```python
from build123d import *

# Parameters (mm, degrees)
SKETCH1_R           = 15
BOSS_EXTRUDE1_DEPTH = 10
SKETCH2_R           = 3.75
CUT_EXTRUDE1_DEPTH  = 5
SKETCH3_R           = 3.75
CUT_EXTRUDE2_DEPTH  = 24.452078799


with BuildPart() as part:
    # Sketch1 → Boss-Extrude1 (new body)
    with BuildSketch(Plane(origin=(0, 0, 0), x_dir=(1, 0, 0), z_dir=(0, 1, 0))):
        with Locations(Location((0, 0, 0), (0, 0, 270))):
            Circle(SKETCH1_R)
    extrude(amount=BOSS_EXTRUDE1_DEPTH)

    # Sketch2 → Cut-Extrude1 (cut)
    with BuildSketch(Plane.XZ):
        with Locations(Location((0, 0, 0), (0, 0, 270))):
            Circle(SKETCH2_R)
    extrude(amount=-CUT_EXTRUDE1_DEPTH, mode=Mode.SUBTRACT)

    # Sketch3 → Cut-Extrude2 (cut, through all)
    with BuildSketch(Plane(origin=(0, 10, 0), x_dir=(1, 0, 0), z_dir=(0, 1, 0))):
        with Locations(Location((0, 0, 0), (0, 0, 90))):
            Circle(SKETCH3_R)
    extrude(amount=-CUT_EXTRUDE2_DEPTH, mode=Mode.SUBTRACT)


solid = part.part
```
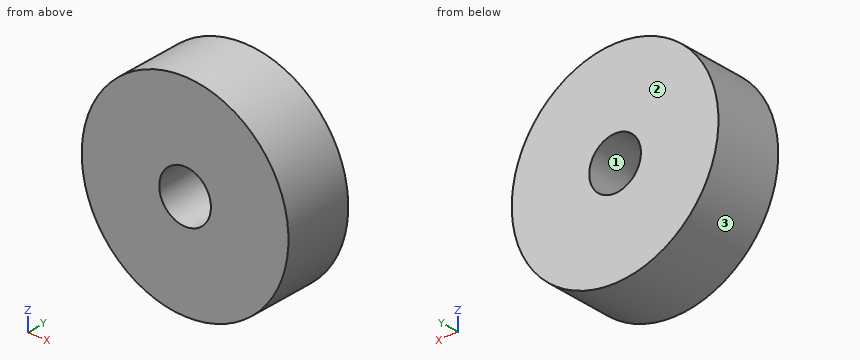
Input: part model. Units: mm. Frame: model coordinates. Face numbers are marked on the shaded views. Give positions to 0.01 mm unless a question says otherwise; leave off trailing zeros. Order: outer loops, then holes, each group sorted by start corner. A loop starts at its lowest first (then second) coordinate and runs counter-clockwise, first axis right, second up. Notation, with made-up numbers: (-22, -16.5) - (-2, -16.5) arc R17 cw to (-2, 16.5) - close; hole circle Ø4 at (85.5, -30). An arc over 180 degrees is marked (long way). Use a Markdown table: item, result.
(1) Line query: line 1 (X direction, y = 3, z = 0); line 2 (X direction, y = 9, z = 1.75); line 3 (X direction, y = 9.5, z = 4.25). Output: solid intervals per line, ascending. Write a range as from..to.
Computed values:
| item | result |
|---|---|
| line 1 | x = -15..-3.75, 3.75..15 |
| line 2 | x = -14.9..-3.32, 3.32..14.9 |
| line 3 | x = -14.39..14.39 |
(2) Pin query (flat end, axial travel): pin 1 (5 mm diameter, centred on y = 6, z = 6, fed in from -X); pin 2 (3 mm diameter, centred on x = 12, y = 9, fed in from -Z); pin 3 (2 mm diameter, centred on x = 10, y = 1, fed in from -Z). Return the tip coordinate at first contact, or that it passes through.
Computed values:
| item | result |
|---|---|
| pin 1 | stops at x = -14.59 |
| pin 2 | stops at z = -10.71 |
| pin 3 | stops at z = -12 |
(3) Draft query along Z for the marked faces 1, 2 and 3. Return one class per face: released by +Z, released by -Z, zero draft, split by the parting line, or undercut.
Computed values:
| item | result |
|---|---|
| face 1 | undercut |
| face 2 | zero draft |
| face 3 | split by the parting line |
(4) Section query D-D (x = -8). Output: boundary loops of the cut face in (y, z), then the cut area to 3 significant figures.
Computed values:
| item | result |
|---|---|
| outline | (0, -12.69) - (10, -12.69) - (10, 12.69) - (0, 12.69) - close |
| area | 254 mm2 |
(5) Section query A-A (x = 0). Output: boundary loops of the cut face in (y, z), then the cut area to 3 significant figures.
Computed values:
| item | result |
|---|---|
| outline | (0, -15) - (10, -15) - (10, -3.75) - (0, -3.75) - close; (0, 3.75) - (10, 3.75) - (10, 15) - (0, 15) - close |
| area | 225 mm2 |
(6) Section query B-B (z = 0). Output: boundary loops of the cut face in (x, y).
Computed values:
| item | result |
|---|---|
| outline | (-15, 0) - (-3.75, 0) - (-3.75, 10) - (-15, 10) - close; (3.75, 0) - (15, 0) - (15, 10) - (3.75, 10) - close |
(7) Section query C-C (y = 5.25). Output: boundary loops of the cut face in (x, z), then the cut area to 3 significant figures.
Computed values:
| item | result |
|---|---|
| outline | circle Ø30 at (0, 0); hole circle Ø7.5 at (0, 0) |
| area | 663 mm2 |
